```python
from build123d import *

# Parameters (mm, degrees)
F0_R     = 5.4
F1_DEPTH = 1.5
F3_DEPTH = 3
F5_DEPTH = 3
F6_R     = 1


with BuildPart() as f1:
    # F0 (on Top) → F1 (new body, symmetric)
    with BuildSketch(Plane.XY):
        Circle(F0_R)
        with BuildLine():
            ThreePointArc((1.525, 2.1057955741), (2.3157072354, 1.1821590418), (2.6, 0))
            ThreePointArc((2.6, 0), (2.3157072354, -1.1821590418), (1.525, -2.1057955741))
            ThreePointArc((1.525, -2.1057955741), (0, -2.6), (-1.525, -2.1057955741))
            ThreePointArc((-1.525, -2.1057955741), (-2.6, 0), (-1.525, 2.1057955741))
            ThreePointArc((-1.525, 2.1057955741), (0, 2.6), (1.525, 2.1057955741))
        make_face(mode=Mode.SUBTRACT)
        with BuildLine():
            ThreePointArc((1.525, -2.1057955741), (2.3157072354, -1.1821590418), (2.6, 0))
            ThreePointArc((2.6, 0), (2.3157072354, 1.1821590418), (1.525, 2.1057955741))
            Line((1.525, 2.1057955741), (1.525, -2.1057955741))
        make_face()
        with BuildLine():
            Line((-1.525, -2.1057955741), (-1.525, 2.1057955741))
            ThreePointArc((-1.525, 2.1057955741), (-2.6, 0), (-1.525, -2.1057955741))
        make_face()
    extrude(amount=F1_DEPTH, both=True)

    # F2 (on face) → F3 (join, through all)
    with BuildSketch(Plane.XY.offset(1.5)):
        with BuildLine():
            ThreePointArc((-2, 5.0159744816), (0, 5.4), (2, 5.0159744816))
            Line((2, 5.0159744816), (3.0470652436, 35))
            Line((3.0470652436, 35), (0, 35))
            Line((0, 35), (-3.0470652436, 35))
            Line((-3.0470652436, 35), (-2, 5.0159744816))
        make_face()
    extrude(amount=-F3_DEPTH)

    # F4 (on face) → F5 (join, through all)
    with BuildSketch(Plane.XY.offset(1.5)):
        Polygon((0, 47.5), (-7.5, 35), (-3.0470652436, 35), (3.0470652436, 35), (7.5, 35), align=None)
    extrude(amount=-F5_DEPTH)

    # F6
    f6_edges = [f1.edges().sort_by_distance(p)[0] for p in [
        (-7.5, 35, 0),
        (0, 47.5, 0),
        (7.5, 35, 0),
    ]]
    fillet(f6_edges, radius=F6_R)


solid = f1.part
```
Verification items for the finished model (mm, model axes). A direction names the side the tool comes from. Coordinates: 2 decimals unless noted, no trailing zeros. Write each loop counter-clockwise with the first axis right and the second up, starting at its lowest first coordinate (ties: lowest second). Pieces come first, ordered by that corner, then holes. Notation, with made-up numbers: M 11.25,8 L 56.25,8 A18 ccw 56.25,40 Z; hole C -27,-9.5 d8. An arc over 180 degrees is marked long. One line per item, written item: value.
Item 1: Section check B-B, the plane z = -0.3. Record the boundary of the cut face in (x, y) (1 decimal).
Check sheet entries:
outline: M -6.6,36.5 A1 ccw -5.7,35 L -3,35 L -2,5 A5.4 ccw long 2,5 L 3,35 L 5.7,35 A1 ccw 6.6,36.5 L 0.9,46.1 A1 ccw -0.9,46.1 Z; hole M -1.5,-2.1 A2.6 ccw 1.5,-2.1 L 1.5,2.1 A2.6 ccw -1.5,2.1 Z
Item 2: Scan lines: line 1 along Y through (x, z) = (-4.25, -1.2); line 2 along X through (y, z) = (-1, -0.15) (3 decimals); line 3 along Y through (x, z) = (4.5, -0.4). Record each from-to range of solid material in increasing order.
Check sheet entries:
line 1: y = -3.33 to 3.33, 35 to 40.42
line 2: x = -5.307 to -1.525, 1.525 to 5.307
line 3: y = -2.98 to 2.98, 35 to 40
Item 3: Access from +Z, -Z, +X, -X, +Y, -Y to the whole of each face (thin tool, end or side, straight path). Record for faces 4 (the flat face through (-4, 35, 0)), 5 (the flat face through (4, 35, 0)), 6 (the flat face through (1.525, 0, 0)).
Check sheet entries:
face 4: +Z, -Z, -X
face 5: +Z, -Z, +X
face 6: +Z, -Z
Item 4: Gauge pin test, flat ends, axial feed: pin 1 Ø1 at (x, y) = (-3, 7.5) entering from +Z; pin 2 Ø0.9 at (y, z) = (1, 0.5) entering from +X; pin 3 Ø1.5 at (x, z) = (5, -1) entering from +Y; pin 4 Ø1.5 at (y, z) = (1, 0) entering from -X. Record the tip position at first contact, or that the pin passes through.
Check sheet entries:
pin 1: passes through
pin 2: stops at x = 5.37
pin 3: stops at y = 40.42
pin 4: stops at x = -5.39
Item 5: Section check C-C, the plane y = 0. Record the boundary of the cut face in (x, z) (3 decimals), plus the area to 4 significant figures.
Check sheet entries:
outline: M -5.4,-1.5 L -1.525,-1.5 L -1.525,1.5 L -5.4,1.5 Z; M 1.525,-1.5 L 5.4,-1.5 L 5.4,1.5 L 1.525,1.5 Z
area: 23.25 mm^2
Item 6: Mould release check, pull along X, two halves, no side actions. Record for faces 1 (the cylindrical face through (0, -2.6, 0)), 2 (the flat face through (0, 21, 1.5)), 3 (the cylindrical face through (-0.209, -5.396, 0.021)): pulls with the +X half, pulls with the -X half, needs draft (parallel to the pull), parting line crosses it, or undercut.
Check sheet entries:
face 1: undercut
face 2: needs draft
face 3: parting line crosses it
Item 7: Section check D-D, the plane y = 8. Record the boundary of the cut face in (x, z).
Check sheet entries:
outline: M -2.1,-1.5 L 2.1,-1.5 L 2.1,1.5 L -2.1,1.5 Z
Item 8: Section check A-A, the plane x = 0. Record the boundary of the cut face in (y, z).
Check sheet entries:
outline: M -5.4,-1.5 L -2.6,-1.5 L -2.6,1.5 L -5.4,1.5 Z; M 2.6,-1.5 L 46.56,-1.5 L 46.56,1.5 L 2.6,1.5 Z
